Geometry check sheet. Reference: the model listing, model coordinates, mm. Face numbers are marked on the shaded views. A direction names the side the tool comes from. Coordinates: 2 decimals unless noted, no trailing zeros. Write each loop counter-clockwise with the first axis right and the second up, starting at its lowest first coordinate (ties: lowest second). Pieces come first, ordered by that corner, then holes. Notation, with made-up numbers: (77.25, 29) -> (85.25, 29) arc R11 ccw to (85.25, 49) -> close; hole circle Ø10 at (64.25, -17.5). An arc over 180 degrees is marked (long way). Answer as CSV lines item,"result".
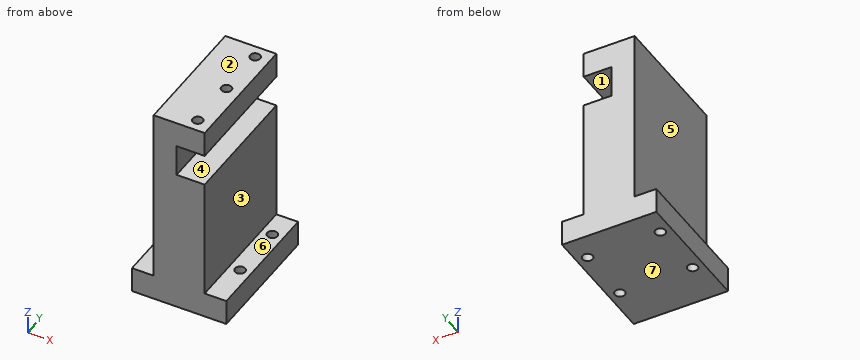
```python
from build123d import *

# Parameters (mm, degrees)
SZKIC1_W                    = 74
SZKIC1_H                    = 100
DODANIE_WYCI_GNI_CIE1_DEPTH = 20
SZKIC3_W                    = 40
SZKIC3_H                    = 100
DODANIE_WYCI_GNI_CIE2_DEPTH = 140
SZKIC4_R                    = 4
WYTNIJ_WYCI_GNI_CIE1_DEPTH  = 20
SZYK_LINIOWY1_COUNT         = 2
SZYK_LINIOWY1_PITCH         = 45
SZYK_LINIOWY1_COUNT_DIR2    = 2
SZYK_LINIOWY1_PITCH_DIR2    = 57
SZKIC5_W                    = 22
SZKIC5_H                    = 25
WYTNIJ_WYCI_GNI_CIE2_DEPTH  = 100
SZKIC6_R                    = 4
WYTNIJ_WYCI_GNI_CIE3_DEPTH  = 10


with BuildPart() as part:
    # Szkic1 → Dodanie-wyciągnięcie1 (new body)
    with BuildSketch(Plane.XY):
        Rectangle(SZKIC1_W, SZKIC1_H)
    extrude(amount=DODANIE_WYCI_GNI_CIE1_DEPTH)

    # Szkic3 → Dodanie-wyciągnięcie2 (add)
    with BuildSketch(Plane.XY.offset(20)):
        Rectangle(SZKIC3_W, SZKIC3_H)
    extrude(amount=DODANIE_WYCI_GNI_CIE2_DEPTH)

    # Szkic4 → Wytnij-wyciągnięcie1 (cut)
    with BuildSketch(Plane.XY.offset(20)):
        with Locations((-28.5, 29.3)):
            Circle(SZKIC4_R)
    wytnij_wyci_gni_cie1 = extrude(amount=-WYTNIJ_WYCI_GNI_CIE1_DEPTH, mode=Mode.SUBTRACT)

    # Szyk liniowy1: Wytnij-wyci_gni_cie1 2 × 2
    with Locations(*[(j * SZYK_LINIOWY1_PITCH_DIR2, -i * SZYK_LINIOWY1_PITCH, 0) for i in range(SZYK_LINIOWY1_COUNT) for j in range(SZYK_LINIOWY1_COUNT_DIR2) if (i, j) != (0, 0)]):
        add(wytnij_wyci_gni_cie1, mode=Mode.SUBTRACT)

    # Szkic5 → Wytnij-wyciągnięcie2 (cut)
    with BuildSketch(Plane(origin=(0, 50, 0), x_dir=(1, 0, 0), z_dir=(0, 1, 0))):
        with Locations((9, -127.5)):
            Rectangle(SZKIC5_W, SZKIC5_H)
    extrude(amount=-WYTNIJ_WYCI_GNI_CIE2_DEPTH, mode=Mode.SUBTRACT)

    # Szkic6 → Wytnij-wyciągnięcie3 (cut)
    with BuildSketch(Plane.XY.offset(160)):
        with Locations((9, 40)):
            Circle(SZKIC6_R)
        with Locations((9, 0)):
            Circle(SZKIC6_R)
        with Locations((9, -40)):
            Circle(SZKIC6_R)
    extrude(amount=-WYTNIJ_WYCI_GNI_CIE3_DEPTH, mode=Mode.SUBTRACT)


solid = part.part
```
Item 1: Thickness scan on probe 1 along Y at (x, z) = (28, 4); probe 2 along Y at (x, z) = (9, 153); probe 3 along X at (y, z) = (29, 13). Record the ranges inside material, lowest first.
Responses:
probe 1,"y = -50 to -19.67, -11.73 to 25.33, 33.27 to 50"
probe 2,"y = -50 to -44, -36 to -4, 4 to 36, 44 to 50"
probe 3,"x = -37 to -32.49, -24.51 to 24.51, 32.49 to 37"
Item 2: Cross-section at D-D, the plane z = 18. Record the cut outline in (x, y).
Responses:
outline,"(-37, -50) -> (37, -50) -> (37, 50) -> (-37, 50) -> close; hole circle Ø8 at (-28.5, -15.7); hole circle Ø8 at (-28.5, 29.3); hole circle Ø8 at (28.5, -15.7); hole circle Ø8 at (28.5, 29.3)"
Item 3: Depth check by flat-ended pin: pin 1 Ø13.5 at (x, y) = (31, -14) entering from +Z; pin 2 Ø10 at (y, z) = (26, 65.5) entering from -X; pin 3 Ø22 at (y, z) = (-8, 151) entering from +X. Enter the tip coordinate at first touch or a pass-through.
Responses:
pin 1,"stops at z = 20"
pin 2,"stops at x = -20"
pin 3,"stops at x = 20"
Item 4: Release check for a two-part mould opening along Z. For the marked faces 1, 2 and 3 record: +Z half, -Z half, draft (parallel to the pull), parting line (faces both ways), or undercut.
Responses:
face 1,"undercut"
face 2,"+Z half"
face 3,"draft"
Item 5: Cross-section at C-C, the plane x = 28.5. Record the cut outline in (y, z).
Responses:
outline,"(-50, 0) -> (-19.7, 0) -> (-19.7, 20) -> (-50, 20) -> close; (-11.7, 0) -> (25.3, 0) -> (25.3, 20) -> (-11.7, 20) -> close; (33.3, 0) -> (50, 0) -> (50, 20) -> (33.3, 20) -> close"
Item 6: Set-up check for the marked faces 4, 5, 6 and 7: record each of +Z, -Z, +X, -X, +Y, -Y from which the full face is reachable in a straight line by a thin tool's end or side.
Responses:
face 4,"+X, +Y, -Y"
face 5,"+Z, -X, +Y, -Y"
face 6,"+Z, +X, +Y, -Y"
face 7,"-Z, +X, -X, +Y, -Y"
Item 7: Cross-section at A-A, the plane x = 9. Record the cut outline in (y, z).
Responses:
outline,"(-50, 0) -> (50, 0) -> (50, 115) -> (-50, 115) -> close; (-50, 140) -> (50, 140) -> (50, 160) -> (44, 160) -> (44, 150) -> (36, 150) -> (36, 160) -> (4, 160) -> (4, 150) -> (-4, 150) -> (-4, 160) -> (-36, 160) -> (-36, 150) -> (-44, 150) -> (-44, 160) -> (-50, 160) -> close"
Item 8: Cross-section at B-B, the plane y = -15.7. Record the cut outline in (x, z).
Responses:
outline,"(-37, 0) -> (-32.5, 0) -> (-32.5, 20) -> (-37, 20) -> close; (-24.5, 0) -> (24.5, 0) -> (24.5, 20) -> (20, 20) -> (20, 115) -> (-2, 115) -> (-2, 140) -> (20, 140) -> (20, 160) -> (-20, 160) -> (-20, 20) -> (-24.5, 20) -> close; (32.5, 0) -> (37, 0) -> (37, 20) -> (32.5, 20) -> close"
